Here's how the part is built. I have some questions about the finished solid (model axes, mm). A direction names the side the tool comes from. Round coordinates to 2 decimals unless told otherwise and drop trailing zeros. Write each loop counter-clockwise with the first axis right and the second up, starting at its lowest first coordinate (ties: lowest second). Pieces come first, ordered by that corner, then holes. Notation, with made-up numbers: M 75,15.25 L 103,15.25 A36 ccw 103,52.25 Z; hole C 56,85.25 d10. An arc over 180 degrees is marked long. Write item = value, one per line. Start each with the question number.
(1) I want a section at C-C (y = 10). List the corners of the cut face in (x, z) for me, and give its area (3 significant figures).
(2) I want a section at B-B (x = 14). List the corners of the cut face in (y, z) for me.
(3) I need wall thicknesses on line 1 along Y through (x, z) = (10, 5.5); line 2 along Y through (x, z) = (10, 8.25); line 3 along X through (y, z) = (29.5, 11). Which ranges of each line are inside material? Lowest first, please.
(4) I want a section at A-A (z = 10). List the corners of the cut face in (x, y) for me, and give its area (3 significant figures).
(5) I want a section at D-D (x = 30). List the corners of the cut face in (y, z) for me.
(6) On a 3-axis mill with a long thin cutter (end or side, diameter ignored), from which of +Z, -Z, +X, -X, +Y, -Y can I reach the whole of each face in a straight line? I mean faces 5 (the flat face through (20, 55, 8)), 6 (the flat face through (17.001, 20, 11)), 7 (the flat face through (40, 35, 5)). Say none if no direction works.
(7) If we mould it in two halves opening along X, with no side actions, what happens to faces 1 (the flat face through (19, 20, 9)), 2 (the flat face through (20, 70, 4)), 3 (the cylindrical face through (1.711, 68.196, 4.056)), 4 (the cylindrical face through (25.733, 47.033, 4.056))? For each: released by +X, released by -X, zero draft, split by the parting line, or undercut.
(8) Will these pins go through, and if not, where does the flat tip stop? pin 1 Ø2 at (x, z) = (24.5, 10) entering from +Y; pin 2 Ø1.5 at (x, y) = (20, 25.5) entering from +Z; pin 3 Ø3.5 at (x, y) = (14, 45) entering from -Z; pin 4 Ø15 at (x, y) = (13, 48.5) entering from +Z.
```python
from build123d import *

# Parameters (mm, degrees)
SKETCH_W        = 40
SKETCH_H        = 70
SKETCH_R        = 2.6
PAD_DEPTH       = 12
SKETCH001_W     = 40
SKETCH001_H     = 30
POCKET_DEPTH    = 4
SKETCH002_R     = 2.05
POCKET001_DEPTH = 10
SKETCH003_W     = 5
SKETCH003_H     = 40.063374
POCKET002_DEPTH = 3
FILLET_R        = 6


with BuildPart() as part:
    # Sketch → Pad (new body)
    with BuildSketch(Plane.XY):
        with Locations((20, 35)):
            Rectangle(SKETCH_W, SKETCH_H)
        with Locations((10, 10)):
            Circle(SKETCH_R, mode=Mode.SUBTRACT)
        with Locations((30, 10)):
            Circle(SKETCH_R, mode=Mode.SUBTRACT)
        with Locations((10, 30)):
            Circle(SKETCH_R, mode=Mode.SUBTRACT)
        with Locations((30, 30)):
            Circle(SKETCH_R, mode=Mode.SUBTRACT)
    extrude(amount=PAD_DEPTH)

    # Sketch001 (on Face10 of Pad) → Pocket (cut)
    with BuildSketch(Plane.XY.offset(12)):
        with Locations((20, 55)):
            Rectangle(SKETCH001_W, SKETCH001_H)
    extrude(amount=-POCKET_DEPTH, mode=Mode.SUBTRACT)

    # Sketch002 (on Face7 of Pocket) → Pocket001 (cut)
    with BuildSketch(Plane.XY.offset(8)):
        with Locations((14, 45)):
            Circle(SKETCH002_R)
        with Locations((26, 45)):
            Circle(SKETCH002_R)
    extrude(amount=-POCKET001_DEPTH, mode=Mode.SUBTRACT)

    # Sketch003 (on Face5 of Pocket001) → Pocket002 (cut)
    with BuildSketch(Plane.XY.offset(12)):
        with Locations((19.500526, 20.031687)):
            Rectangle(SKETCH003_W, SKETCH003_H)
    extrude(amount=-POCKET002_DEPTH, mode=Mode.SUBTRACT)

    # Fillet
    fillet_edges = [part.edges().sort_by_distance(p)[0] for p in [
        (40, 0, 6),
        (40, 70, 4),
        (0, 70, 4),
        (0, 0, 6),
    ]]
    fillet(fillet_edges, radius=FILLET_R)


solid = part.part
```
Returned:
q1.outline = M 0,0 L 7.4,0 L 7.4,12 L 0,12 Z; M 12.6,0 L 27.4,0 L 27.4,12 L 22,12 L 22,9 L 17,9 L 17,12 L 12.6,12 Z; M 32.6,0 L 40,0 L 40,12 L 32.6,12 Z
q1.area = 340 mm²
q2.outline = M 0,0 L 42.95,0 L 42.95,8 L 40,8 L 40,12 L 0,12 Z; M 47.05,0 L 70,0 L 70,8 L 47.05,8 Z
q3.line_1 = 0 to 7.4, 12.6 to 27.4, 32.6 to 70
q3.line_2 = 0 to 7.4, 12.6 to 27.4, 32.6 to 40
q3.line_3 = 0 to 7.45, 12.55 to 17, 22 to 27.45, 32.55 to 40
q4.outline = M 0,6 A6 ccw 6,0 L 17,0 L 17,40 L 0,40 Z; M 22,0 L 34,0 A6 ccw 40,6 L 40,40 L 22,40 Z; hole C 10,10 d5.2; hole C 10,30 d5.2; hole C 30,10 d5.2; hole C 30,30 d5.2
q4.area = 1,300 mm²
q5.outline = M 0,0 L 7.4,0 L 7.4,12 L 0,12 Z; M 12.6,0 L 27.4,0 L 27.4,12 L 12.6,12 Z; M 32.6,0 L 70,0 L 70,8 L 40,8 L 40,12 L 32.6,12 Z
q6.face_5 = +Z, +X, -X, +Y
q6.face_6 = +Z, +Y, -Y
q6.face_7 = +Z, -Z, +X, +Y, -Y
q7.face_1 = undercut
q7.face_2 = zero draft
q7.face_3 = released by -X
q7.face_4 = undercut
q8.pin_1 = 40
q8.pin_2 = 9
q8.pin_3 = through
q8.pin_4 = 8
